Geometry check sheet. Reference: the model listing, model coordinates, mm. A direction names the side the tool comes from. Coordinates: 2 decimals unless noted, no trailing zeros. Write each loop counter-clockwise with the first axis right and the second up, starting at its lowest first coordinate (ties: lowest second). Pieces come first, ordered by that corner, then holes. Notation, with made-up numbers: (-8.75, 27.5) -> (25.25, 27.5) arc R18 cw to (25.25, 35.5) -> close; hole circle Ø5 at (73, 87.25). An arc over 180 degrees is marked (long way). One line per question, with ' | ' between items.
from build123d import *

# Parameters (mm, degrees)
ESQUISSE1_W                               = 42
ESQUISSE1_H                               = 42
BOSS_EXTRU_1_DEPTH                        = 48
CHANFREIN1_SIZE                           = 2
ESQUISSE3_R                               = 13
BOSS_EXTRU_2_DEPTH                        = 3
TROU_POUR_TARAUDAGE_POUR_TROU_TARAUD_M3_D = 2.5
ESQUISSE7_R                               = 2.5
BOSS_EXTRU_3_DEPTH                        = 22
CHANFREIN2_SIZE                           = 0.4
CHANFREIN3_SIZE                           = 0.4
ENL_V_START                               = -9
ENL_V_MAT_EXTRU_1_DEPTH                   = 30


with BuildPart() as part:
    # Esquisse1 → Boss.-Extru.1 (new body)
    with BuildSketch(Plane.XY):
        Rectangle(ESQUISSE1_W, ESQUISSE1_H)
    extrude(amount=BOSS_EXTRU_1_DEPTH)

    # Chanfrein1
    chanfrein1_edges = [part.edges().sort_by_distance(p)[0] for p in [
        (-21, 21, 24),
        (21, 21, 24),
        (21, -21, 24),
        (-21, -21, 24),
    ]]
    chamfer(chanfrein1_edges, length=CHANFREIN1_SIZE)

    # Esquisse3 → Boss.-Extru.2 (add)
    with BuildSketch(Plane.XY.offset(48)):
        Circle(ESQUISSE3_R)
    extrude(amount=BOSS_EXTRU_2_DEPTH)

    # Trou pour taraudage pour trou taraudé M3x0.51 (through all)
    with Locations(Plane.XY.offset(48)):
        with Locations((-15.5, 15.5), (-15.5, -15.5), (15.5, -15.5), (15.5, 15.5)):
            Hole(TROU_POUR_TARAUDAGE_POUR_TROU_TARAUD_M3_D / 2)

    # Esquisse7 → Boss.-Extru.3 (add)
    with BuildSketch(Plane.XY.offset(51)):
        Circle(ESQUISSE7_R)
    extrude(amount=BOSS_EXTRU_3_DEPTH)

    # Chanfrein2
    chanfrein2_edges = [part.edges().sort_by_distance(p)[0] for p in [
        (-2.5, 0, 73),
    ]]
    chamfer(chanfrein2_edges, length=CHANFREIN2_SIZE)

    # Chanfrein3
    chanfrein3_edges = [part.edges().sort_by_distance(p)[0] for p in [
        (-13, 0, 51),
    ]]
    chamfer(chanfrein3_edges, length=CHANFREIN3_SIZE)

    # Esquisse9 → Enlèv. mat.-Extru.1 (cut)
    with BuildSketch(Plane(origin=(0, 0, 0), x_dir=(-1, 0, 0), z_dir=(0, 0, -1)).offset(ENL_V_START)):
        Polygon((-21, 15), (-15, 21), (-21, 21), align=None)
        Polygon((15, 21), (21, 15), (21, 21), align=None)
        Polygon((-21, -15), (-15, -21), (-21, -21), align=None)
        Polygon((15, -21), (21, -15), (21, -21), align=None)
    extrude(amount=-ENL_V_MAT_EXTRU_1_DEPTH, mode=Mode.SUBTRACT)


solid = part.part
1. Tool access check on faces 1 (the face through (-19, -19, 9)), 2 (the face through (19, -19, 9)), 3 (the face through (-19, 19, 39)), 4 (the face through (19, 19, 9)). Record the directions out of +Z, -Z, +X, -X, +Y, -Y that give a thin tool (end or side, any length) a straight path to the whole face; none if there is none.
Worked answers:
face 1: -X, -Y | face 2: +X, -Y | face 3: -X, +Y | face 4: +X, +Y
2. Cross-section at D-D on z = 17.5. Record the boundary of the cut face in (x, y), and give its area (3 significant figures).
Worked answers:
outline: (-21, -15) -> (-15, -21) -> (15, -21) -> (21, -15) -> (21, 15) -> (15, 21) -> (-15, 21) -> (-21, 15) -> close; hole circle Ø2.5 at (-15.5, -15.5); hole circle Ø2.5 at (-15.5, 15.5); hole circle Ø2.5 at (15.5, -15.5); hole circle Ø2.5 at (15.5, 15.5) | area: 1,670 mm²
3. Cross-section at A-A on z = 40. Record the boundary of the cut face in (x, y).
Worked answers:
outline: (-21, -19) -> (-19, -21) -> (19, -21) -> (21, -19) -> (21, 19) -> (19, 21) -> (-19, 21) -> (-21, 19) -> close; hole circle Ø2.5 at (-15.5, -15.5); hole circle Ø2.5 at (-15.5, 15.5); hole circle Ø2.5 at (15.5, -15.5); hole circle Ø2.5 at (15.5, 15.5)
4. Cross-section at B-B on x = 0. Record the boundary of the cut face in (y, z).
Worked answers:
outline: (-21, 0) -> (21, 0) -> (21, 48) -> (13, 48) -> (13, 50.6) -> (12.6, 51) -> (2.5, 51) -> (2.5, 72.6) -> (2.1, 73) -> (-2.1, 73) -> (-2.5, 72.6) -> (-2.5, 51) -> (-12.6, 51) -> (-13, 50.6) -> (-13, 48) -> (-21, 48) -> close
5. Material ranges on line 1 (Y direction, x = -15.5, z = 24); line 2 (Y direction, x = -16, z = 19.5); line 3 (X direction, y = -15, z = 30), recorded low to high. Write a range as from..to.
Worked answers:
line 1: -20.5..-16.75, -14.25..14.25, 16.75..20.5 | line 2: -20..-16.65, -14.35..14.35, 16.65..20 | line 3: -21..-16.65, -14.35..14.35, 16.65..21
6. Mould release check, pull along Y, two halves, no side actions. Record for faces 5 (the face through (0, 0, 73)), 6 (the face through (-15.34, -14.26, 23.66)), 7 (the face through (-20, -20, 43)): released by +Y, released by -Y, zero draft, split by the parting line, or undercut.
Worked answers:
face 5: zero draft | face 6: undercut | face 7: released by -Y
7. Go/stop test with flat-tipped pins: P1, Ø1.8, axis at x = -17.5, y = 16.5, coming from the +Z side; P2, Ø2, axis at x = -15.5, y = -15.5, coming from the +Z side. Record where each tip stops, or that it passes through.
Worked answers:
P1: z = 48 | P2: through
